Here's how the part is built. I have some questions about the finished solid (model axes, mm). A direction names the side the tool comes from. Round coordinates to 2 decimals unless told otherwise and drop trailing zeros. Order: outer loops, then holes, each group sorted by start corner. A loop starts at its lowest first (then second) coordinate and runs counter-clockwise, first axis right, second up. Notation, with made-up numbers: M 25.5,57 L 84.5,57 A26 cw 84.5,77 Z; hole C 10,-22.5 d3. An arc over 180 degrees is marked long. Use one line per item in the form item = value. Start each with the question number.
```python
from build123d import *

# Parameters (mm, degrees)
BOSS_EXTRUDE1_DEPTH = 1
EXTRUDE_THIN1_START = 1
EXTRUDE_THIN1_DEPTH = 0.2


with BuildPart() as part:
    # Sketch3 → Boss-Extrude1 (new body)
    with BuildSketch(Plane(origin=(0, 0, 0), x_dir=(1, 0, 0), z_dir=(0, 1, 0))):
        with BuildLine():
            Line((143.614236161, 12.778644367), (143.614236161, 6.690833444))
            Line((143.614236161, 6.690833444), (83.614236161, 6.690833444))
            Line((83.614236161, 6.690833444), (68.614236161, 6.690833444))
            ThreePointArc((68.614236161, 6.690833444), (75.180479735, 23.997298156), (71.779240838, 42.192375773))
            ThreePointArc((71.779240838, 42.192375773), (51.379079295, 63.12072091), (24.905577059, 75.502800726))
            ThreePointArc((24.905577059, 75.502800726), (11.315687886, 83.748123559), (5.247844857, 98.440016471))
            ThreePointArc((5.247844857, 98.440016471), (7.693142423, 109.618807389), (15.866887418, 117.62722417))
            ThreePointArc((15.866887418, 117.62722417), (96.637810578, 139.573762678), (179.070811064, 125.068832083))
            ThreePointArc((179.070811064, 125.068832083), (185.95529686, 120.311391566), (190.290589438, 113.153555076))
            Line((190.290589438, 113.153555076), (190.62158299, 112.199107439))
            ThreePointArc((190.62158299, 112.199107439), (191.44765289, 108.968802746), (191.725584387, 105.646151098))
            Line((191.725584387, 105.646151098), (191.725584387, 88.676044486))
            ThreePointArc((191.725584387, 88.676044486), (190.474138078, 74.473395816), (185.740302271, 61.024524277))
            ThreePointArc((185.740302271, 61.024524277), (167.758196388, 34.211461518), (143.614236161, 12.778644367))
        make_face()
    extrude(amount=BOSS_EXTRUDE1_DEPTH)

    # Sketch6 → Extrude-Thin1 (add)
    with BuildSketch(Plane(origin=(0, 0, 0), x_dir=(1, 0, 0), z_dir=(0, 1, 0)).offset(EXTRUDE_THIN1_START)):
        with BuildLine():
            ThreePointArc((135.157565874, 25.167539704), (156.459213519, 44.077209645), (172.324402154, 67.73374361))
            ThreePointArc((172.324402154, 67.73374361), (175.840861474, 77.773394532), (176.725584387, 88.374212526))
            Line((176.725584387, 88.374212526), (176.725584387, 105.646151098))
            ThreePointArc((176.725584387, 105.646151098), (175.822683582, 108.923695738), (173.313645893, 111.217657072))
            ThreePointArc((173.313645893, 111.217657072), (97.321055557, 124.589331548), (22.860686061, 104.357454747))
            ThreePointArc((22.860686061, 104.357454747), (20.817249813, 102.355350552), (20.205925421, 99.560652822))
            ThreePointArc((20.205925421, 99.560652822), (22.75737939, 93.448802044), (28.458504402, 90.078073505))
            ThreePointArc((28.458504402, 90.078073505), (60.346877221, 75.148921347), (84.753788625, 49.770769703))
            ThreePointArc((84.753788625, 49.770769703), (90.951279239, 28.051793518), (83.614236161, 6.690833444))
            Line((83.614236161, 6.690833444), (83.45325287, 6.809511075))
            ThreePointArc((83.45325287, 6.809511075), (90.751349173, 28.057082078), (84.586756318, 49.660768756))
            ThreePointArc((84.586756318, 49.660768756), (60.232106569, 74.985116949), (28.412138365, 89.883479249))
            ThreePointArc((28.412138365, 89.883479249), (22.605157011, 93.319061801), (20.006484347, 99.545711004))
            ThreePointArc((20.006484347, 99.545711004), (20.642261714, 102.452196643), (22.767435413, 104.534385006))
            ThreePointArc((22.767435413, 104.534385006), (97.315220897, 124.789273275), (173.396463183, 111.39982251))
            ThreePointArc((173.396463183, 111.39982251), (175.99119074, 109.031493114), (176.925584387, 105.644975177))
            Line((176.925584387, 105.644975177), (176.925584387, 88.378563485))
            ThreePointArc((176.925584387, 88.378563485), (176.036009323, 77.729553344), (172.503280822, 67.644287353))
            ThreePointArc((172.503280822, 67.644287353), (156.609866623, 43.945666337), (135.270321477, 25.002354432))
            Line((135.270321477, 25.002354432), (135.157565874, 25.167539704))
        make_face()
        Polygon((143.614236161, 6.690833444), (124.886408885, 47.608659456), (125.068265889, 47.691894244), (143.796093165, 6.774068232), align=None)
    extrude(amount=EXTRUDE_THIN1_DEPTH)


solid = part.part
```
1) If I drill on line 1 (Y direction, x = 110, z = -111.5); line 2 (X direction, y = 0.55, z = -101.5); line 3 (Z direction, x = 22.5, y = 1.15), over which ranges is the centre line in solid material (lowest first)?
2) If we mould it in two halves opening along Z, with no side actions, what happens to faces 3 (the flat face through (117, 1, -80)), 4 (the cylindrical face through (185.87, 0.49, -120.4)), 5 (the cylindrical face through (75.156, 0.493, -23.736)), 6 (the flat face through (100, 0, -74))? For each: +Z half, -Z half, draft (parallel to the pull), parting line (faces both ways), or undercut.
3) Will these pins go through, and if not, where does the flat tip stop? pin 1 Ø0.5 at (y, z) = (0.5, -8.5) entering from +X; pin 2 Ø5 at (x, z) = (120.5, -87) entering from +Y.
4) If we section it at B-B on z = -38.5: Write out the boundary of the cut face in (x, y), then the cut area to 3 significant figures.
5) If we section it at A-A on y = 0.4: Write out the boundary of the cut face in (x, z), then the cut area to 3 significant figures.
6) If we section it at C-C on x = 167: Write out the boundary of the cut face in (y, z), then the cut area to 3 significant figures.
7) On a 3-axis mill with a long thin cutter (end or side, diameter ignored), from which of +Z, -Z, +X, -X, +Y, -Y can I reach the whole of each face in a straight line? I mean faces 1 (the flat face through (99, 1, -128)), 2 (the cylindrical face through (95.458, 0.493, -139.516)). Say none if no direction works.
8) If we section it at D-D on x = 118: Write out the boundary of the cut face in (y, z).
Completed:
q1.line_1 = 0 to 1
q1.line_2 = 5.25 to 191.73
q1.line_3 = -104.38 to -104.15, -93.76 to -93.44
q2.face_3 = undercut
q2.face_4 = -Z half
q2.face_5 = undercut
q2.face_6 = draft
q3.pin_1 = 143.61
q3.pin_2 = 1
q4.outline = M 73.34,0 L 171.34,0 L 171.34,1 L 151.53,1 L 151.53,1.2 L 151.25,1.2 L 151.25,1 L 129.28,1 L 129.28,1.2 L 129.06,1.2 L 129.06,1 L 89.76,1 L 89.76,1.2 L 89.55,1.2 L 89.55,1 L 73.34,1 Z
q4.area = 98.1 mm²
q5.outline = M 5.25,-98.44 A20 ccw 15.87,-117.63 A191.99 ccw 179.07,-125.07 A20 ccw 190.29,-113.15 L 190.62,-112.2 A20 ccw 191.73,-105.65 L 191.73,-88.68 A57.05 ccw 185.74,-61.02 A127.42 ccw 143.61,-12.78 L 143.61,-6.69 L 68.61,-6.69 A34.24 cw 71.78,-42.19 A81.47 cw 24.91,-75.5 A25.51 ccw Z
q5.area = 17,600 mm²
q6.outline = M 0,-129.62 L 1,-129.62 L 1,-113.91 L 1.2,-113.91 L 1.2,-113.7 L 1,-113.7 L 1,-58.26 L 1.2,-58.26 L 1.2,-57.89 L 1,-57.89 L 1,-33.35 L 0,-33.35 Z
q6.area = 96.4 mm²
q7.face_1 = +Y
q7.face_2 = -Z, +Y, -Y
q8.outline = M 0,-139.36 L 1,-139.36 L 1,-124.52 L 1.2,-124.52 L 1.2,-124.32 L 1,-124.32 L 1,-6.69 L 0,-6.69 Z
